```python
from build123d import *

# Parameters (mm, degrees)
F1_DEPTH        = 533.4
F3_DEPTH        = 25.4
F5_DEPTH        = 25.4
F7_DEPTH        = 25.4
F8_W            = 127
F8_H            = 139.7
F10_DEPTH       = 25.4
F13_D           = 20.32
F13_DEPTH       = 50.8
F13_CBORE_D     = 27.94
F13_CBORE_DEPTH = 5.08
F13_TIP         = 6.1047438893
F14_R           = 6.35
F15_DEPTH       = 5.08
F16_R           = 2.54
F17_DEPTH       = 5.08
F18_R           = 2.54
F19_DEPTH       = 5.08
F20_R           = 2.54
F21_DEPTH       = 5.08
F22_R           = 2.54
F23_DEPTH       = 5.08
F25_DEPTH       = 533.4


with BuildPart() as f1:
    # F0 (on Front) → F1 (new body)
    with BuildSketch(Plane.XZ):
        Polygon((73.373222708, 160.7664102355), (-155.226777292, 160.7664102355), (-155.226777292, 66.7864102355), (-153.6675693713, 51.0384102355), (-129.826777292, 51.0384102355), (-129.826777292, -189.7535897645), (47.973222708, -189.7535897645), (47.973222708, 51.0384102355), (71.8140147872, 51.0384102355), (73.373222708, 66.7864102355), align=None)
        Polygon((-129.826777292, 51.0384102355), (-153.6675693713, 51.0384102355), (-129.826777292, -189.7535897645), align=None)
        Polygon((47.973222708, -189.7535897645), (71.8140147872, 51.0384102355), (47.973222708, 51.0384102355), align=None)
    extrude(amount=F1_DEPTH)

    # F2 (on face) → F3 (cut)
    with BuildSketch(Plane.XZ.offset(533.4)):
        Polygon((-129.826777292, 66.7864102355), (-155.226777292, 66.7864102355), (-129.826777292, -189.7535897645), align=None)
    extrude(amount=-F3_DEPTH, mode=Mode.SUBTRACT)

    # F4 (on face) → F5 (cut)
    with BuildSketch(Plane.XZ.offset(533.4)):
        Polygon((47.973222708, 66.7864102355), (47.973222708, -189.7535897645), (73.373222708, 66.7864102355), align=None)
    extrude(amount=-F5_DEPTH, mode=Mode.SUBTRACT)

    # F6 (on face) → F7 (cut)
    with BuildSketch(Plane(origin=(0, 0, 0), x_dir=(-1, 0, 0), z_dir=(0, 1, 0))):
        Polygon((-47.973222708, 66.7864102355), (-73.373222708, 66.7864102355), (-47.973222708, -189.7535897645), align=None)
        Polygon((129.826777292, 66.7864102355), (129.826777292, -189.7535897645), (155.226777292, 66.7864102355), align=None)
    extrude(amount=-F7_DEPTH, mode=Mode.SUBTRACT)

    # F8 (on face) → F10 (cut)
    with BuildSketch(Plane(origin=(0, 0, -189.7535897645), x_dir=(1, 0, 0), z_dir=(0, 0, -1))):
        with Locations((-40.926777292, 95.25)):
            Rectangle(F8_W, F8_H)
    extrude(amount=-F10_DEPTH, mode=Mode.SUBTRACT)

    # F13
    with Locations(Plane(origin=(0, 0, -164.3535897645), x_dir=(1, 0, 0), z_dir=(0, 0, -1))):
        with Locations((-40.926777292, 95.25)):
            CounterBoreHole(F13_D / 2, F13_CBORE_D / 2, F13_CBORE_DEPTH, depth=F13_DEPTH)
            with Locations((0, 0, -(F13_DEPTH + F13_TIP / 2))):  # 118° drill point
                Cone(0, F13_D / 2, F13_TIP, mode=Mode.SUBTRACT)

    # F14 (on offset) → F15 (join)
    with BuildSketch(Plane(origin=(0, 0, -164.3535897645), x_dir=(1, 0, 0), z_dir=(0, 0, -1))):
        with Locations((-40.926777292, 132.08)):
            Circle(F14_R)
        with Locations((-40.926777292, 58.42)):
            Circle(F14_R)
    extrude(amount=F15_DEPTH)

    # F16 (on face) → F17 (join)
    with BuildSketch(Plane(origin=(0, 0, 66.7864102355), x_dir=(1, 0, 0), z_dir=(0, 0, -1))):
        with Locations((60.673222708, 12.7)):
            Circle(F16_R)
    extrude(amount=F17_DEPTH)

    # F18 (on face) → F19 (join)
    with BuildSketch(Plane(origin=(0, 0, 66.7864102355), x_dir=(1, 0, 0), z_dir=(0, 0, -1))):
        with Locations((-141.6487544775, 12.7)):
            Circle(F18_R)
    extrude(amount=F19_DEPTH)

    # F20 (on face) → F21 (join)
    with BuildSketch(Plane(origin=(0, 0, 66.7864102355), x_dir=(1, 0, 0), z_dir=(0, 0, -1))):
        with Locations((60.673222708, 520.7)):
            Circle(F20_R)
    extrude(amount=F21_DEPTH)

    # F22 (on face) → F23 (join)
    with BuildSketch(Plane(origin=(0, 0, 66.7864102355), x_dir=(1, 0, 0), z_dir=(0, 0, -1))):
        with Locations((-142.526777292, 520.7)):
            Circle(F22_R)
    extrude(amount=F23_DEPTH)

    # F24 (on face) → F25 (join)
    with BuildSketch(Plane(origin=(0, 0, 0), x_dir=(-1, 0, 0), z_dir=(0, 1, 0))):
        with BuildLine():
            Line((-73.373222708, 160.7664102355), (155.226777292, 160.7664102355))
            ThreePointArc((155.226777292, 160.7664102355), (40.926777292, 176.1690639423), (-73.373222708, 160.7664102355))
        make_face()
    extrude(amount=-F25_DEPTH)


solid = f1.part
```
Read the model definition and answer for the solid it produces. Units are mm, in the model's axes. A direction names the side the tool comes from. Coordinates: 2 decimals unless noted, no trailing zeros. Order: outer loops, then holes, each group sorted by start corner. A loop starts at its lowest first (then second) coordinate and runs counter-clockwise, first axis right, second up. Notation, with made-up numbers: (-2, 37.25) - (15, 37.25) arc R20 ccw to (15, 67.25) - close; hole circle Ø5 at (73, 64). An arc over 180 degrees is marked (long way). Answer as a JSON object with one key per item and string values. Group by question number.
Item 1: Flat-ended cylindrical pins translate along their axes: P1, Ø4, axis at x = -42.5, y = -58.5, coming from the -Z side; P2, Ø2, axis at y = -412, z = -24.5, coming from the -X side; P3, Ø1.5, axis at x = -128, y = -334, coming from the +Z side. Find the tip coordinate at first contact, or state that the pin passes through.
Item 2: The mould has two halves that part along Y. Classify faces 3 (the face through (-155.227, -263, 114)), 4 (the face through (-39, -533.4, -4)), 5 (the face through (-33.42, -107.03, -161.85)): +Y half, -Y half, draft (parallel to the pull), parting line (faces both ways), or undercut.
Item 3: Section B-B (z = 9) is taken. Give the vertices of the cut face in (x, y), plus the area to 3 significant figures.
Item 4: Section A-A (y = -132.08) is taken. Give the vertices of the cut face in (x, z).
Item 5: Section D-D (x = -72) is taken. Give the vertices of the cut face in (y, z), plus the area to 3 significant figures.
Item 6: Consider probe 1 along Z at (x, y) = (-40.5, -51); probe 2 along X at (y, z) = (-70, -170); probe 3 along X at (y, z) = (-95.25, -160.4). Determine where each line is inside the solid, lowest interval first. Write a range as from..to.
Item 7: A tool of negligible diameter and unlimited length cuts with its end or side. For faces 1 (the face through (-35.06, -129.65, -166.86)), 2 (the face through (-42, -322, -189.754)), from which of +Z, -Z, +X, -X, +Y, -Y can it reach the whole face along a straight path? Write none if from no direction.
Item 8: Section C-C (z = -128) is taken. Give the vertices of the cut face in (x, y), plus the area to 3 significant figures.
Results are:
{
 "1": {"P1": "stops at z = -169.43", "P2": "stops at x = -146.29", "P3": "stops at z = 167.45"},
 "2": {"face 3": "draft", "face 4": "-Y half", "face 5": "undercut"},
 "3": {"outline": "(-149.51, -508) - (-129.83, -508) - (-129.83, -533.4) - (47.97, -533.4) - (47.97, -508) - (67.65, -508) - (67.65, -25.4) - (47.97, -25.4) - (47.97, 0) - (-129.83, 0) - (-129.83, -25.4) - (-149.51, -25.4) - close", "area": "114,000 mm^2"},
 "4": {"outline": "(-155.23, 66.79) - (-129.83, -189.75) - (-104.43, -189.75) - (-104.43, -164.35) - (-47.28, -164.35) - (-47.28, -169.43) - (-34.58, -169.43) - (-34.58, -164.35) - (22.57, -164.35) - (22.57, -189.75) - (47.97, -189.75) - (73.37, 66.79) - (73.37, 160.77) arc R431.8 ccw to (-155.23, 160.77) - close"},
 "5": {"outline": "(-533.4, -189.75) - (-165.1, -189.75) - (-165.1, -164.35) - (-25.4, -164.35) - (-25.4, -189.75) - (0, -189.75) - (0, 175.05) - (-533.4, 175.05) - close", "area": "191,000 mm^2"},
 "6": {"probe 1": "z = -164.35..176.17", "probe 2": "x = -131.78..-104.43, 22.57..49.93", "probe 3": "x = -132.73..-54.9, -26.96..50.88"},
 "7": {"face 1": "-Z", "face 2": "-Z, +X, -X, +Y, -Y"},
 "8": {"outline": "(-135.94, -508) - (-129.83, -508) - (-129.83, -533.4) - (47.97, -533.4) - (47.97, -508) - (54.09, -508) - (54.09, -25.4) - (47.97, -25.4) - (47.97, 0) - (-129.83, 0) - (-129.83, -25.4) - (-135.94, -25.4) - close; hole circle Ø20.32 at (-40.93, -95.25)", "area": "100,000 mm^2"}
}
